Could you check a few things on this model? Use its own coordinates, in mm. A direction names the side the tool comes from. Round coordinates to 2 decimals unless told otherwise and drop trailing zeros. Write each loop counter-clockwise with the first axis right and the second up, starting at its lowest first coordinate (ties: lowest second). Pieces come first, ordered by that corner, then holes. Notation, with made-up numbers: (6, 89) -> (62, 89) arc R22 cw to (62, 119) -> close; hole circle Ø4 at (6, 55). An arc over 180 degrees is marked (long way). Answer in a Markdown table with one row per item.
from build123d import *

# Parameters (mm, degrees)
SKETCH_R        = 17.5
PAD_DEPTH       = 50
SKETCH001_R     = 9.5
POCKET_DEPTH    = 18.5
SKETCH002_R     = 5
POCKET001_DEPTH = 18.5


with BuildPart() as part:
    # Sketch → Pad (new body)
    with BuildSketch(Plane.XZ):
        Circle(SKETCH_R)
    extrude(amount=PAD_DEPTH)

    # Sketch001 (on Face3 of Pad) → Pocket (cut)
    with BuildSketch(Plane.XZ.offset(50)):
        Circle(SKETCH001_R)
    extrude(amount=-POCKET_DEPTH, mode=Mode.SUBTRACT)

    # Sketch002 (on Face2 of Pocket) → Pocket001 (cut)
    with BuildSketch(Plane(origin=(0, 0, 0), x_dir=(1, 0, 0), z_dir=(0, 1, 0))):
        Circle(SKETCH002_R)
    extrude(amount=-POCKET001_DEPTH, mode=Mode.SUBTRACT)


solid = part.part
1) Thinking about a two-plate mould opening in Z: for faces 1 (the face through (8, -50, -8)), 2 (the face through (-13.887, -24.65, -10.648)), 3 (the face through (-1.08, -9.12, 4.88)), which applies, +Z half, -Z half, draft (parallel to the pull), parting line (faces both ways), or undercut?
Findings:
| item | result |
|---|---|
| face 1 | draft |
| face 2 | parting line |
| face 3 | undercut |
2) Imagine slicing it at A-A, the plane y = -4.5. Please give me the cut outline in (x, z).
Findings:
| item | result |
|---|---|
| outline | circle Ø35 at (0, 0); hole circle Ø10 at (0, 0) |
3) For pin 1 (5 mm diameter, centred on x = -4.5, z = -8, fed in from -Y); pin 2 (1 mm diameter, centred on y = -40, z = 9.5, fed in from +X); pin 3 (10 mm diameter, centred on y = -6, z = 11, fed in from -X); pin 4 (3 mm diameter, centred on x = -1, z = 0, fed in from +Y), each with a flat end and sliding along its axis, tell me the tip position at first contact or that it passes through.
Findings:
| item | result |
|---|---|
| pin 1 | stops at y = -50 |
| pin 2 | stops at x = 15.01 |
| pin 3 | stops at x = -16.44 |
| pin 4 | stops at y = -18.5 |
4) For faces 4 (the face through (0, -18.5, 0)), 5 (the face through (4, 0, -4)), 6 (the face through (0, -31.5, 0)), which set-ups out of +Z, -Z, +X, -X, +Y, -Y let a thin tool reach every point of the face, with its end or its side?
Findings:
| item | result |
|---|---|
| face 4 | +Y |
| face 5 | +Z, -Z, +X, -X, +Y |
| face 6 | -Y |
5) Imagine slicing it at C-C, the plane x = 0. Please give me the cut outline in (y, z).
Findings:
| item | result |
|---|---|
| outline | (-50, -17.5) -> (0, -17.5) -> (0, -5) -> (-18.5, -5) -> (-18.5, 5) -> (0, 5) -> (0, 17.5) -> (-50, 17.5) -> (-50, 9.5) -> (-31.5, 9.5) -> (-31.5, -9.5) -> (-50, -9.5) -> close |
6) Imagine slicing it at D-D, the plane z = 7. Please give me the cut outline in (x, y), plus the area to 3 significant figures.
Findings:
| item | result |
|---|---|
| outline | (-16.04, -50) -> (-6.42, -50) -> (-6.42, -31.5) -> (6.42, -31.5) -> (6.42, -50) -> (16.04, -50) -> (16.04, 0) -> (-16.04, 0) -> close |
| area | 1,370 mm^2 |
7) Please list where these lines run through material, in increasing order: line 1 (Z direction, x = 0, y = -45.25); line 2 (Z direction, x = 0, y = -8.5); line 3 (Y direction, x = 3.5, z = 3.5).
Findings:
| item | result |
|---|---|
| line 1 | z = -17.5 to -9.5, 9.5 to 17.5 |
| line 2 | z = -17.5 to -5, 5 to 17.5 |
| line 3 | y = -31.5 to -18.5 |
8) Imagine slicing it at B-B, the plane z = 0. Please give me the cut outline in (x, y), plus the area to 3 significant figures.
Findings:
| item | result |
|---|---|
| outline | (-17.5, -50) -> (-9.5, -50) -> (-9.5, -31.5) -> (9.5, -31.5) -> (9.5, -50) -> (17.5, -50) -> (17.5, 0) -> (5, 0) -> (5, -18.5) -> (-5, -18.5) -> (-5, 0) -> (-17.5, 0) -> close |
| area | 1,210 mm^2 |
